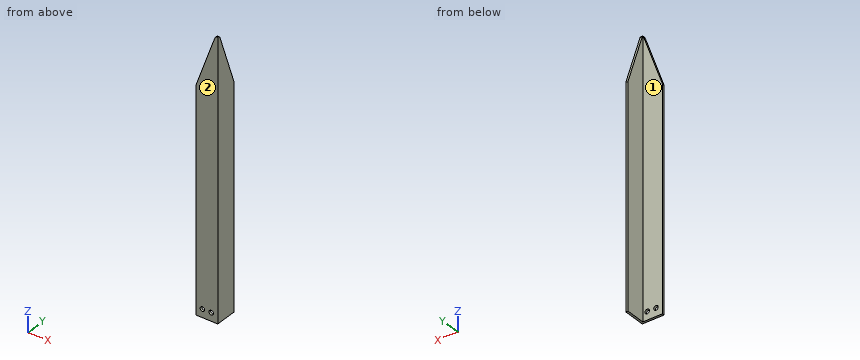
```python
from build123d import *

# Parameters (mm, degrees)
EXTRUDE_1_DEPTH     = 250
CUT_EXTRUDE_1_DEPTH = 10
CUT_EXTRUDE_2_DEPTH = 10
FILLET_1_R          = 3
SKETCH_5_R          = 2.05
CUT_EXTRUDE_4_DEPTH = 10


with BuildPart() as part:
    # 草图1 → 凸台-拉伸1 (new body)
    with BuildSketch(Plane.XY):
        Polygon((-20, 0), (0, 0), (0, 20), (-2, 20), (-2, 2), (-20, 2), align=None)
    extrude(amount=EXTRUDE_1_DEPTH)

    # 草图2 → 切除-拉伸1 (cut)
    with BuildSketch(Plane.ZY.offset(2)):
        Polygon((250, 2), (200, 20), (250, 20), align=None)
    extrude(amount=-CUT_EXTRUDE_1_DEPTH, mode=Mode.SUBTRACT)

    # 草图3 → 切除-拉伸2 (cut)
    with BuildSketch(Plane(origin=(0, 2, 0), x_dir=(1, 0, 0), z_dir=(0, 1, 0))):
        Polygon((-2, -250), (-20, -200), (-20, -250), align=None)
    extrude(amount=-CUT_EXTRUDE_2_DEPTH, mode=Mode.SUBTRACT)

    # 圆角1
    # the kernel refuses this fillet: 3 mm, written as the material it takes off along each edge
    with BuildSketch(Plane(origin=(-7.265916136, 2, 250), x_dir=(0, -1, 0), z_dir=(1, 0, 0))) as fillet_1_piece_1:
        with BuildLine():
            CenterArc((2.10919491, 2.998012087), FILLET_1_R, 199.798876355, 68.115193721)
            Line((-0.713467325, 1.981853682), (-0.76992057, 1.961530514))
            Line((-0.76992057, 1.961530514), (-0.056453245, -0.020323168))
            Line((-0.056453245, -0.020323168), (0, -0.06))
            ThreePointArc((0, -0.06), (1, -0.06), (1.997816102, -0.059960242))
            Line((1.997816102, -0.059960242), (2, 0))
        make_face()
    extrude(amount=12.531832272, mode=Mode.SUBTRACT)
    with BuildSketch(Plane(origin=(-2, 7.265916136, 250), x_dir=(1, 0, 0), z_dir=(0, -1, 0))) as fillet_1_piece_2:
        with BuildLine():
            CenterArc((2.10919491, -2.998012087), FILLET_1_R, 92.085929924, 68.115193721)
            Line((-0.713467325, -1.981853682), (-0.76992057, -1.961530514))
            Line((-0.76992057, -1.961530514), (-0.056453245, 0.020323168))
            Line((-0.056453245, 0.020323168), (0, 0.06))
            ThreePointArc((0, 0.06), (1, 0.06), (1.997816102, 0.059960242))
            Line((1.997816102, 0.059960242), (2, 0))
        make_face()
    extrude(amount=12.531832272, mode=Mode.SUBTRACT)

    # 草图5 → 切除-拉伸4 (cut)
    with BuildSketch(Plane.XZ):
        with Locations(Location((-14, 7.5, 0), (0, 0, 270))):
            Circle(SKETCH_5_R)
        with Locations(Location((-6, 7.5, 0), (0, 0, 270))):
            Circle(SKETCH_5_R)
    extrude(amount=-CUT_EXTRUDE_4_DEPTH, mode=Mode.SUBTRACT)


solid = part.part
```
CAD build for the part. Positions are in the model's coordinates, mm. Face numbers are marked on the shaded views. A direction names the side the tool comes from. Round coordinates to 2 decimals unless told otherwise and drop trailing zeros. Order: outer loops, then holes, each group sorted by start corner. A loop starts at its lowest first (then second) coordinate and runs counter-clockwise, first axis right, second up. Notation, with made-up numbers: (-27.5, 86.25) -> (22.5, 86.25) arc R27 ccw to (22.5, 113.25) -> close; hole circle Ø4 at (-5, 7.5). An arc over 180 degrees is marked (long way). Write item = value, one per line.
(1) 3-axis set-ups, long thin cutter, end or side, ignore diameter. For the marked faces 1 and 2: which of +Z, -Z, +X, -X, +Y, -Y reach the whole face in a straight line?
Answers follow:
face_1 = +Z, -Z, -X, +Y
face_2 = +Z, -Z, +X, -X, -Y
(2) Cut at B-B (x = -6). Write the cut outline in (y, z), plus the area to 3 significant figures.
Answers follow:
outline = (0, 0) -> (2, 0) -> (2, 5.45) -> (0, 5.45) -> close; (0, 9.55) -> (2, 9.55) -> (2, 238.89) -> (0, 238.89) -> close
area = 470 mm²
(3) Cut at C-C (z = 78). Write the cut outline in (x, y).
Answers follow:
outline = (-20, 0) -> (0, 0) -> (0, 20) -> (-2, 20) -> (-2, 2) -> (-20, 2) -> close
(4) Flat gauge pins, fed straight in: P1, Ø8, axis at y = 14.5, z = 212, coming from the -X side; P2, Ø2.5, axis at x = -14, z = 7.5, coming from the +Y side. Where does each tip first touch, or does it go through?
Answers follow:
P1 = -2
P2 = through
(5) Cut at A-A (z = 7.5). Write the cut outline in (x, y).
Answers follow:
outline = (-20, 0) -> (-16.05, 0) -> (-16.05, 2) -> (-20, 2) -> close; (-11.95, 0) -> (-8.05, 0) -> (-8.05, 2) -> (-11.95, 2) -> close; (-3.95, 0) -> (0, 0) -> (0, 20) -> (-2, 20) -> (-2, 2) -> (-3.95, 2) -> close
(6) Drill centre lines: L1, parallel to X at y = 1, z = 7.5; L2, parallel to Y at x = -3.5, z = 152.5; L3, parallel to X at y = 2.5, z = 106. Where is each one in solid material? Low to high.
Answers follow:
L1 = -20 to -16.05, -11.95 to -8.05, -3.95 to 0
L2 = 0 to 2
L3 = -2 to 0
(7) Cut at D-D (y = 6.5). Write the cut outline in (x, z), plus the area to 3 significant figures.
Answers follow:
outline = (-2, 0) -> (0, 0) -> (0, 237.5) -> (-2, 237.5) -> close
area = 475 mm²
